Read the model definition and answer for the solid it produces. Units are mm, in the model's axes. Face numbers are marked on the shaded views. A direction names the side the tool comes from. Give positions to 0.01 mm unless a question says otherwise; leave off trailing zeros. Order: outer loops, then holes, each group sorted by start corner. A loop starts at its lowest first (then second) coordinate and runs counter-clockwise, first axis right, second up.
```python
from build123d import *

# Parameters (mm, degrees)
SKETCH_1_W          = 198
SKETCH_1_H          = 298
SKETCH_1_W_2        = 175
SKETCH_1_H_2        = 275
EXTRUDE_1_DEPTH     = 80
SKETCH_2_W          = 198
SKETCH_2_H          = 298
EXTRUDE_2_DEPTH     = 3.5
SKETCH_3_W          = 200
SKETCH_3_H          = 300
SKETCH_3_W_2        = 194
SKETCH_3_H_2        = 294
CUT_EXTRUDE_1_DEPTH = 25


with BuildPart() as part:
    # 草图1 → 凸台-拉伸1 (new body)
    with BuildSketch(Plane(origin=(0, 0, 0), x_dir=(1, 0, 0), z_dir=(0, 1, 0))):
        Rectangle(SKETCH_1_W, SKETCH_1_H)
        Rectangle(SKETCH_1_W_2, SKETCH_1_H_2, mode=Mode.SUBTRACT)
    extrude(amount=-EXTRUDE_1_DEPTH)

    # 草图2 → 凸台-拉伸2 (add)
    with BuildSketch(Plane(origin=(0, 0, 0), x_dir=(1, 0, 0), z_dir=(0, 1, 0))):
        Rectangle(SKETCH_2_W, SKETCH_2_H)
    extrude(amount=EXTRUDE_2_DEPTH)

    # 草图3 → 切除-拉伸1 (cut, symmetric)
    with BuildSketch(Plane(origin=(0, -40, 0), x_dir=(-1, 0, 0), z_dir=(0, -1, 0))):
        Rectangle(SKETCH_3_W, SKETCH_3_H)
        Rectangle(SKETCH_3_W_2, SKETCH_3_H_2, mode=Mode.SUBTRACT)
    extrude(amount=CUT_EXTRUDE_1_DEPTH, both=True, mode=Mode.SUBTRACT)


solid = part.part
```
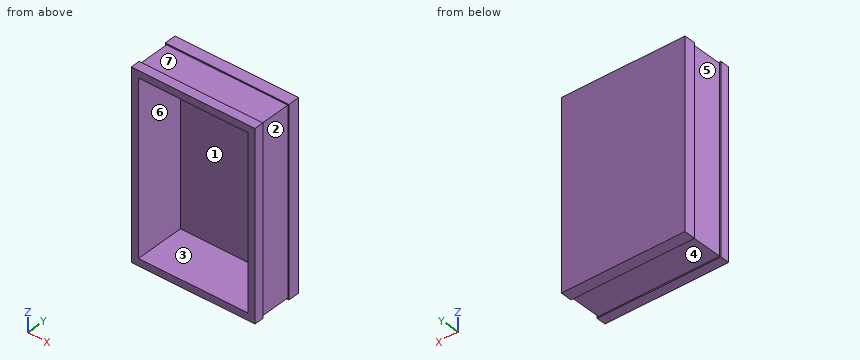
1) The part is cut by section C-C on z = 43. Determine the outline of the cut face in (x, y).
Final values:
outline: (-99, -80) - (-87.5, -80) - (-87.5, 0) - (87.5, 0) - (87.5, -80) - (99, -80) - (99, -65) - (97, -65) - (97, -15) - (99, -15) - (99, 3.5) - (-99, 3.5) - (-99, -15) - (-97, -15) - (-97, -65) - (-99, -65) - close
2) For a pull along Y with two mould halves and no side action, classify the marked faces 1, 2 and 3 as released by +Y, released by -Y, zero draft, split by the parting line, or undercut.
Final values:
face 1: released by -Y
face 2: undercut
face 3: zero draft
3) Consider L1, parallel to Z at x = 3.5, y = -1.5; L2, parallel to X at y = -53, z = -27; L3, parallel to X at y = -7.5, z = -89. Determine where each line is inside the solid, lowest interval first.
Final values:
L1: z = -149 to -137.5, 137.5 to 149
L2: x = -97 to -87.5, 87.5 to 97
L3: x = -99 to -87.5, 87.5 to 99
4) The part is cut by section B-B on x = -78. Determine the outline of the cut face in (y, z), and give its area (3 significant figures).
Final values:
outline: (-80, -149) - (-65, -149) - (-65, -147) - (-15, -147) - (-15, -149) - (3.5, -149) - (3.5, 149) - (-15, 149) - (-15, 147) - (-65, 147) - (-65, 149) - (-80, 149) - (-80, 137.5) - (0, 137.5) - (0, -137.5) - (-80, -137.5) - close
area: 2,680 mm2
5) The part is cut by section A-A on y = -6.5. Determine the outline of the cut face in (x, z).
Final values:
outline: (-99, -149) - (99, -149) - (99, 149) - (-99, 149) - close; hole (-87.5, -137.5) - (87.5, -137.5) - (87.5, 137.5) - (-87.5, 137.5) - close
6) The part is cut by section D-D on y = -44.5. Determine the outline of the cut face in (x, z).
Final values:
outline: (-97, -147) - (97, -147) - (97, 147) - (-97, 147) - close; hole (-87.5, -137.5) - (87.5, -137.5) - (87.5, 137.5) - (-87.5, 137.5) - close
7) Given pin 1 (6 mm diameter, centred on y = -23, z = -105.5, fed in from -X); pin 2 (24 mm diameter, centred on y = -28, z = 65.5, fed in from +X); pin 3 (4 mm diameter, centred on x = -59, y = -44, fed in from +Z), each flat-ended and moving along its own axis, determine where each tip first touches the part or whether it passes through.
Final values:
pin 1: stops at x = -97
pin 2: stops at x = 97
pin 3: stops at z = 147
8) A tool of negligible diameter and unlimited length cuts with its end or side. For the marked faces 4, 5, 6 and 7, from which of +Z, -Z, +X, -X, +Y, -Y can it reach the whole face along a straight path? Write none if from no direction.
Final values:
face 4: -Z, +X, -X
face 5: +Z, -Z, -X
face 6: -Y
face 7: +Z, +X, -X
